from build123d import *

# Parameters (mm, degrees)
PAD020_DEPTH    = 1
PAD021_DEPTH    = 17
POCKET014_DEPTH = 16
POCKET015_DEPTH = 11.6
SKETCH036_R     = 4
SKETCH036_R_2   = 1.95
SKETCH036_R_3   = 2
PAD022_DEPTH    = 5.5
SKETCH037_R     = 1.95
POCKET016_DEPTH = 8
PAD023_DEPTH    = 2.7
POCKET017_DEPTH = 17


with BuildPart() as part:
    # Sketch032 → Pad020 (new body)
    with BuildSketch(Plane.XY):
        with BuildLine():
            Line((-49.75, 45), (-49.75, -45))
            ThreePointArc((-49.75, -45), (-49.457107, -45.707107), (-48.75, -46))
            Line((-48.75, -46), (48.75, -46))
            ThreePointArc((48.75, -46), (49.457107, -45.707107), (49.75, -45))
            Line((49.75, -45), (49.75, 45))
            ThreePointArc((49.75, 45), (49.457107, 45.707107), (48.75, 46))
            Line((48.75, 46), (-48.75, 46))
            ThreePointArc((-48.75, 46), (-49.457107, 45.707107), (-49.75, 45))
        make_face()
    extrude(amount=PAD020_DEPTH)

    # Sketch033 → Pad021 (join)
    with BuildSketch(Plane.XY):
        with BuildLine():
            Line((-49.75, 45), (-49.75, -45))
            ThreePointArc((-49.75, -45), (-49.457107, -45.707107), (-48.75, -46))
            Line((-48.75, -46), (48.75, -46))
            ThreePointArc((48.75, -46), (49.457107, -45.707107), (49.75, -45))
            Line((49.75, -45), (49.75, 45))
            ThreePointArc((49.75, 45), (49.457107, 45.707107), (48.75, 46))
            Line((48.75, 46), (-48.75, 46))
            ThreePointArc((-48.75, 46), (-49.457107, 45.707107), (-49.75, 45))
        make_face()
        Polygon((-47.75, 34), (-47.75, 21.8), (-8.75, 21.8), (-8.75, -38), (47.75, -38), (47.75, 34), align=None, mode=Mode.SUBTRACT)
    extrude(amount=PAD021_DEPTH)

    # Sketch034 (on Face14 of Pad021) → Pocket014 (cut)
    with BuildSketch(Plane.XY.offset(17)):
        with BuildLine():
            Line((-48.75, 45), (-48.75, 44))
            Line((-48.75, 44), (-10, 44))
            ThreePointArc((-8.5, 42.5), (-8.93934, 43.56066), (-10, 44))
            Line((-8.5, 42.5), (-8.5, 34))
            Line((-8.5, 34), (-7, 34))
            Line((-7, 34), (-7, 42.5))
            ThreePointArc((-5.5, 44), (-6.56066, 43.56066), (-7, 42.5))
            Line((-5.5, 44), (33.25, 44))
            Line((33.25, 44), (33.25, 37.5))
            Line((33.25, 37.5), (40.25, 37.5))
            Line((40.25, 37.5), (40.25, 34))
            Line((41.75, 34), (40.25, 34))
            Line((41.75, 37.5), (41.75, 34))
            Line((41.75, 37.5), (46.25, 37.5))
            Line((46.25, 37.5), (46.25, 34))
            Line((46.25, 34), (48.75, 34))
            Line((48.75, 45), (48.75, 34))
            Line((48.75, 45), (-48.75, 45))
        make_face()
    extrude(amount=-POCKET014_DEPTH, mode=Mode.SUBTRACT)

    # Sketch035 (on Face14 of Pocket014) → Pocket015 (cut)
    with BuildSketch(Plane.XY.offset(17)):
        Polygon((-11.794, 18.358), (-47.75, 18.358), (-47.75, -38), (-11.794, -38), (-11.794, -33), (-8.75, -33), (-8.75, 13.358), (-11.794, 13.358), align=None)
    extrude(amount=-POCKET015_DEPTH, mode=Mode.SUBTRACT)

    # Sketch036 → Pad022 (join)
    with BuildSketch(Plane.XY):
        with Locations((37.75, -6)):
            Circle(SKETCH036_R)
        with Locations((37.75, -6)):
            Circle(SKETCH036_R_2, mode=Mode.SUBTRACT)
        with Locations((37.75, -28)):
            Circle(SKETCH036_R)
        with Locations((37.75, -28)):
            Circle(SKETCH036_R_2, mode=Mode.SUBTRACT)
        with Locations((6.75, -17)):
            Circle(SKETCH036_R_3)
    extrude(amount=PAD022_DEPTH)

    # Sketch037 (on Face14 of Pad022) → Pocket016 (cut)
    with BuildSketch(Plane.XY.offset(17)):
        with Locations((-45.75, -42)):
            Circle(SKETCH037_R)
        with Locations((-30, -42)):
            Circle(SKETCH037_R)
        with Locations((30, -42)):
            Circle(SKETCH037_R)
        with Locations((-45.75, 40)):
            Circle(SKETCH037_R)
        with Locations((-30, 40)):
            Circle(SKETCH037_R)
        with Locations((30, 40)):
            Circle(SKETCH037_R)
        with Locations((45.75, -42)):
            Circle(SKETCH037_R)
    extrude(amount=-POCKET016_DEPTH, mode=Mode.SUBTRACT)

    # Sketch038 (on Face4 of Pocket016) → Pad023 (join)
    with BuildSketch(Plane(origin=(0, 0, 0), x_dir=(1, 0, 0), z_dir=(0, 0, -1))):
        with BuildLine():
            Line((-40.500002, -36), (40.499998, -36))
            Line((40.499998, -36), (40.499998, 46))
            Line((48.75, 46), (40.499998, 46))
            ThreePointArc((49.75, 45), (49.457107, 45.707107), (48.75, 46))
            Line((49.75, -36), (49.75, 45))
            ThreePointArc((48.75, -37), (49.457107, -36.707107), (49.75, -36))
            Line((-48.75, -37), (48.75, -37))
            ThreePointArc((-49.75, -36), (-49.457107, -36.707107), (-48.75, -37))
            Line((-49.75, 45), (-49.75, -36))
            ThreePointArc((-48.750005, 46), (-49.457108, 45.707105), (-49.75, 45))
            Line((-48.750005, 46), (-40.500002, 46))
            Line((-40.500002, 46), (-40.500002, -36))
        make_face()
    extrude(amount=PAD023_DEPTH)

    # Sketch039 → Pocket017 (cut)
    with BuildSketch(Plane.XY):
        with BuildLine():
            ThreePointArc((-10, 0.5), (-15, -4.5), (-10, -9.5))
            Line((-10, -9.5), (10, -9.5))
            ThreePointArc((10, -9.5), (15, -4.5), (10, 0.5))
            Line((-10, 0.5), (10, 0.5))
        make_face()
    extrude(amount=POCKET017_DEPTH, mode=Mode.SUBTRACT)


solid = part.part
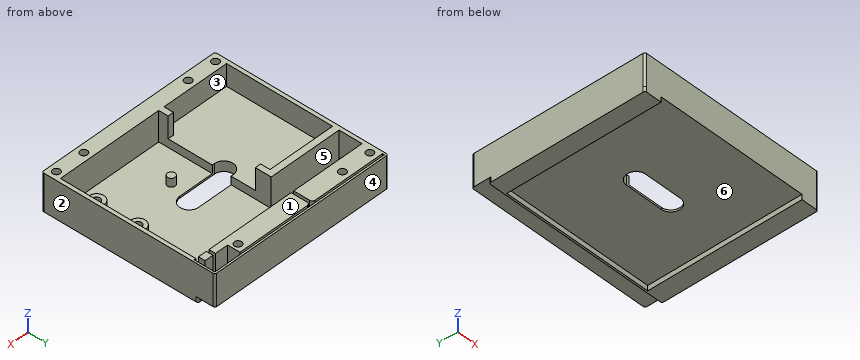
Geometry: final body of the model. Coordinates: model frame, mm. Face numbers are marked on the shaded views. A direction names the side the tool comes from. Give positions to 0.01 mm unless a question says otherwise; leave off trailing zeros. Order: outer loops, then holes, each group sorted by start corner. A loop starts at its lowest first (then second) coordinate and runs counter-clockwise, first axis right, second up. Notation, with made-up numbers: (-29.75, -37) -> (24.25, -37) arc R21 ccw to (24.25, -7) -> close; hole circle Ø1 at (18, 74). An arc over 180 degrees is marked (long way). Answer as a JSON object with one key per item and string values.
Q1. Section D-D (y = -17). Output: boundary loops of the cut face in (x, z), plus the area to 3 significant figures.
Entries:
{"outline": "(-49.75, -2.7) -> (-40.5, -2.7) -> (-40.5, 0) -> (40.5, 0) -> (40.5, -2.7) -> (49.75, -2.7) -> (49.75, 17) -> (47.75, 17) -> (47.75, 1) -> (8.75, 1) -> (8.75, 5.5) -> (4.75, 5.5) -> (4.75, 1) -> (-8.75, 1) -> (-8.75, 5.4) -> (-47.75, 5.4) -> (-47.75, 17) -> (-49.75, 17) -> close", "area": "403 mm^2"}
Q2. Section A-A (y = -42). Output: boundary loops of the cut face in (x, z).
Entries:
{"outline": "(-49.75, -2.7) -> (-40.5, -2.7) -> (-40.5, 0) -> (40.5, 0) -> (40.5, -2.7) -> (49.75, -2.7) -> (49.75, 17) -> (47.7, 17) -> (47.7, 9) -> (43.8, 9) -> (43.8, 17) -> (31.95, 17) -> (31.95, 9) -> (28.05, 9) -> (28.05, 17) -> (-28.05, 17) -> (-28.05, 9) -> (-31.95, 9) -> (-31.95, 17) -> (-43.8, 17) -> (-43.8, 9) -> (-47.7, 9) -> (-47.7, 17) -> (-49.75, 17) -> close"}
Q3. Draft query along X for the marked faces 1, 2 and 3. Return one class per face: released by +X, released by -X, zero draft, split by the parting line, or undercut.
Entries:
{"face 1": "zero draft", "face 2": "released by +X", "face 3": "undercut"}
Q4. Section B-B (x = -45.75). Output: boundary loops of the cut face in (y, z), plus the area to 3 significant figures.
Entries:
{"outline": "(-46, -2.7) -> (37, -2.7) -> (37, 0) -> (46, 0) -> (46, 17) -> (45, 17) -> (45, 1) -> (44, 1) -> (44, 17) -> (41.95, 17) -> (41.95, 9) -> (38.05, 9) -> (38.05, 17) -> (34, 17) -> (34, 1) -> (21.8, 1) -> (21.8, 17) -> (18.36, 17) -> (18.36, 5.4) -> (-38, 5.4) -> (-38, 17) -> (-40.05, 17) -> (-40.05, 9) -> (-43.95, 9) -> (-43.95, 17) -> (-46, 17) -> close", "area": "861 mm^2"}
Q5. Section C-C (z = 14.75). State how many separate pieces and enclosed holes the cut face has, plus the area to 3 significant figures.
Entries:
{"separate pieces": "3", "enclosed holes": "8", "area": "2,130 mm^2"}
Q6. Material intervals for probe 1 along Y at (x, z) = (-45.75, 14); probe 2 along Y at (x, z) = (-28, 14); probe 3 along Y at (x, z) = (39.5, 16.25), sorted ascending.
Entries:
{"probe 1": "y = -46 to -43.95, -40.05 to -38, 18.36 to 21.8, 34 to 38.05, 41.95 to 44, 45 to 46", "probe 2": "y = -46 to -38, 18.36 to 21.8, 34 to 44, 45 to 46", "probe 3": "y = -46 to -38, 34 to 37.5, 45 to 46"}
Q7. Access query for the marked faces 4, 5 and 6. Directions: +Z, -Z, +X, -X, +Y, -Y. A direction counts if a zero-diameter tool reaches every point of the face in a straight line with its end or side. Return the directions, or none.
Entries:
{"face 4": "+Z, -Z, +X, -X, +Y", "face 5": "+Z", "face 6": "-Z, -Y"}
Q8. First-contact query: pin 1 (3 mm diameter, centred on x = -1, y = -8.5, fed in from -Z); pin 2 (5 mm diameter, centred on x = -34, y = 10, fed in from +Z); pin 3 (3 mm diameter, centred on x = 37.75, y = -6, fed in from +Z). Flat tips, straight axial feed; report the tip coordinate or a pass-through.
Entries:
{"pin 1": "stops at z = 0", "pin 2": "stops at z = 5.4", "pin 3": "stops at z = 1"}
